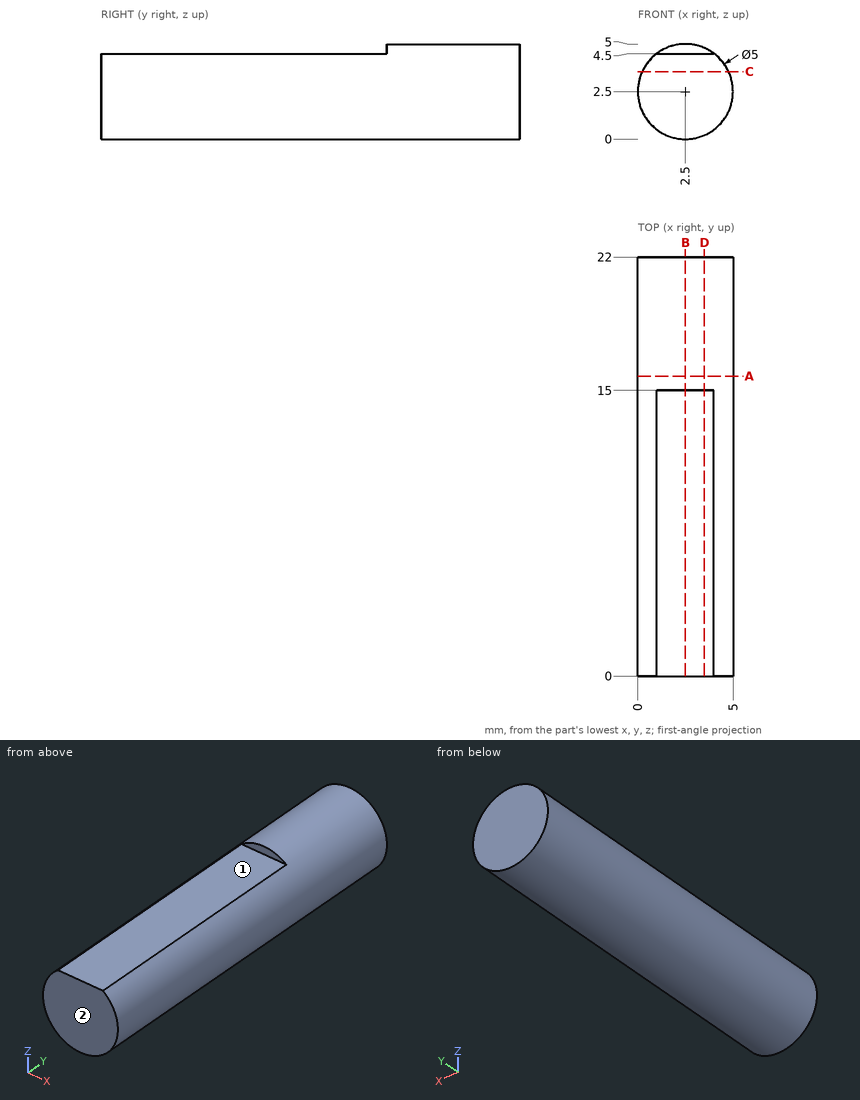
Verification items for this drawing (mm, ordinates from the low corner). A direction names the side the tool comes from. Coordinates: 2 decimals unless noted, no trailing zeros. Write each loop counter-clockwise with the first axis right and the second up, starting at its lowest first coordinate (ties: lowest second). Pieces come first, ordered by that corner, then holes. Notation, with made-up numbers: (4, 29) -> (8, 29) arc R23 ccw to (8, 46) -> close; hole circle Ø4 at (-10.75, 13). An arc over 180 degrees is marked (long way). Use CSV: the item, a comma, the result in double quotes. Start each with the question number.
Item 1: Cross-section at C-C, the plane z = 3.55. Record the cut outline in (x, y).
Item 2: Cross-section at B-B, the plane x = 2.5. Record the cut outline in (y, z), plus the area to 4 significant figures.
Item 3: Depth check by flat-ended pin: pin 1 Ø1 at (y, z) = (12.5, 1.5) entering from +X; pin 2 Ø1.5 at (x, z) = (3.5, 4) entering from -Y; pin 3 Ø1.5 at (x, y) = (4, 5) entering from -Z. Enter the tip coordinate at first touch or a pass-through.
Item 4: Set-up check for the marked faces 1 and 2: record each of +Z, -Z, +X, -X, +Y, -Y from which the full face is reachable in a straight line by a thin tool's end or side.
Item 5: Cross-section at A-A, the plane y = 15.75. Record the cut outline in (x, z), plus the area to 3 significant figures.
Item 6: Thickness scan on line 1 (Z direction, x = 0.5, y = 13.25); line 2 (X direction, y = 1.5, z = 3.95); line 3 (X direction, y = 9.75, z = 1.85). Record the ranges inside material, lowest first.
Item 7: Cross-section at D-D, the plane x = 3.5. Record the cut outline in (y, z).
Answers:
1,outline,"(0.23, 0) -> (4.77, 0) -> (4.77, 22) -> (0.23, 22) -> close"
2,outline,"(0, 0) -> (22, 0) -> (22, 5) -> (15, 5) -> (15, 4.5) -> (0, 4.5) -> close"
2,area,"102.5 mm^2"
3,pin 1,"x = 4.95"
3,pin 2,"y = 0"
3,pin 3,"z = 0.12"
4,face 1,"+Z, +X, -X, -Y"
4,face 2,"+Z, -Z, +X, -X, -Y"
5,outline,"circle Ø5 at (2.5, 2.5)"
5,area,"19.6 mm^2"
6,line 1,"1 to 4"
6,line 2,"0.46 to 4.54"
6,line 3,"0.09 to 4.91"
7,outline,"(0, 0.21) -> (22, 0.21) -> (22, 4.79) -> (15, 4.79) -> (15, 4.5) -> (0, 4.5) -> close"
